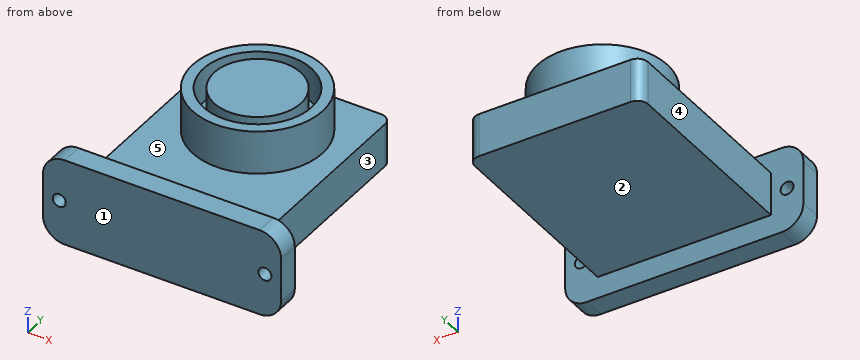
```python
from build123d import *

# Parameters (mm, degrees)
SKETCH1_W           = 40
SKETCH1_H           = 70
BOSS_EXTRUDE1_DEPTH = 10
SKETCH4_R           = 15
BOSS_EXTRUDE3_DEPTH = 10
SKETCH5_R           = 12.5
SKETCH5_R_2         = 10
CUT_EXTRUDE2_DEPTH  = 8
SKETCH6_W           = 40
SKETCH6_H           = 10
CUT_EXTRUDE3_DEPTH  = 17.5
FILLET4_R           = 2.5
SKETCH11_R          = 1.5
SKETCH11_W          = 40
SKETCH11_H          = 10
BOSS_EXTRUDE4_DEPTH = 5


with BuildPart() as part:
    # Sketch1 → Boss-Extrude1 (new body)
    with BuildSketch(Plane.XY):
        Rectangle(SKETCH1_W, SKETCH1_H)
    extrude(amount=BOSS_EXTRUDE1_DEPTH)

    # Sketch4 → Boss-Extrude3 (add)
    with BuildSketch(Plane.XY.offset(10)):
        Circle(SKETCH4_R)
    extrude(amount=BOSS_EXTRUDE3_DEPTH)

    # Sketch5 → Cut-Extrude2 (cut)
    with BuildSketch(Plane.XY.offset(20)):
        Circle(SKETCH5_R)
        Circle(SKETCH5_R_2, mode=Mode.SUBTRACT)
    extrude(amount=-CUT_EXTRUDE2_DEPTH, mode=Mode.SUBTRACT)

    # Sketch6 → Cut-Extrude3 (cut)
    with BuildSketch(Plane(origin=(0, 35, 0), x_dir=(1, 0, 0), z_dir=(0, 1, 0))):
        with Locations((0, -5)):
            Rectangle(SKETCH6_W, SKETCH6_H)
    extrude(amount=-CUT_EXTRUDE3_DEPTH, mode=Mode.SUBTRACT)

    # Fillet4
    fillet4_edges = [part.edges().sort_by_distance(p)[0] for p in [
        (-20, 17.5, 5),
        (20, 17.5, 5),
    ]]
    fillet(fillet4_edges, radius=FILLET4_R)

    # Sketch11 → Boss-Extrude4 (add)
    with BuildSketch(Plane.XZ.offset(35)):
        with BuildLine():
            Line((-22.5, 15), (22.5, 15))
            ThreePointArc((22.5, 15), (26.035533906, 13.535533906), (27.5, 10))
            Line((27.5, 10), (27.5, 0))
            ThreePointArc((27.5, 0), (26.035533906, -3.535533906), (22.5, -5))
            Line((22.5, -5), (-22.5, -5))
            ThreePointArc((-22.5, -5), (-26.035533906, -3.535533906), (-27.5, 0))
            Line((-27.5, 0), (-27.5, 10))
            ThreePointArc((-27.5, 10), (-26.035533906, 13.535533906), (-22.5, 15))
        make_face()
        with Locations((-23.75, 5)):
            Circle(SKETCH11_R, mode=Mode.SUBTRACT)
        with Locations(Location((23.75, 5, 0), (0, 0, 180))):
            Circle(SKETCH11_R, mode=Mode.SUBTRACT)
        with Locations((0, 5)):
            Rectangle(SKETCH11_W, SKETCH11_H, mode=Mode.SUBTRACT)
    extrude(amount=-BOSS_EXTRUDE4_DEPTH)


solid = part.part
```
Can you work these out from the model? Positions are in its coordinate system, mm. Face numbers are marked on the shaded views. A direction names the side the tool comes from. Give positions to 0.01 mm unless a question says otherwise; leave off trailing zeros. Loops run counter-clockwise (first coordinate to the right, second up) from the corner with the lowest first, then second, coordinate; pieces in that order, holes last. Notation, with made-up numbers: M 76.5,24 L 115.5,24 A14 ccw 115.5,48 Z; hole C 72,83.25 d8. An arc over 180 degrees is marked long. One line per question, with ' | ' between items. Start each with the question number.
Q1. For the marked faces 1, 2, 3, 4 and 5, which set-ups out of +Z, -Z, +X, -X, +Y, -Y let a thin tool reach every point of the face, with its end or its side?
Q2. If we section it at D-D (x = -23.75): Please give me the cut outline in (y, z), plus the area to 3 significant figures.
Q3. For pin 1 Ø12 at (x, y) = (5, -11.5) entering from -Z; pin 2 Ø1.5 at (x, y) = (-11, -29) entering from +Z; pin 3 Ø5 at (x, z) = (-23.75, 5) entering from +Y, each with a flat end and sliding along its axis, tell me the tip position at first contact or that it passes through.
Q4. If we section it at C-C (y = -4.5): Please give me the cut outline in (x, z), plus the area to 3 significant figures.
Q5. If we section it at A-A (z = 5): Please give me the cut outline in (x, y).
Q6. If I drill on line 1 (X direction, y = -1.5, z = 4.25); line 2 (Y direction, x = 6.5, z = 14.5); line 3 (Z direction, x = 17, y = 7), over which ranges is the centre line in solid material (lowest first)? Write a range as from..to.
Q7. If we section it at B-B (x = 0): Please give me the cut outline in (y, z).
Computed:
1) face 1: +Z, -Z, +X, -X, -Y | face 2: -Z, +X, -X, +Y | face 3: +Z, -Z, +X, +Y | face 4: +Z, -Z, -X, +Y | face 5: +Z
2) outline: M -35,-4.84 L -30,-4.84 L -30,3.5 L -35,3.5 Z; M -35,6.5 L -30,6.5 L -30,14.84 L -35,14.84 Z | area: 83.4 mm²
3) pin 1: stops at z = 0 | pin 2: stops at z = 10 | pin 3: stops at y = -30
4) outline: M -20,0 L 20,0 L 20,10 L 14.31,10 L 14.31,20 L 11.66,20 L 11.66,12 L 8.93,12 L 8.93,20 L -8.93,20 L -8.93,12 L -11.66,12 L -11.66,20 L -14.31,20 L -14.31,10 L -20,10 Z | area: 642 mm²
5) outline: M -27.5,-35 L -25.25,-35 L -25.25,-30 L -27.5,-30 Z; M -22.25,-35 L 22.25,-35 L 22.25,-30 L 20,-30 L 20,15 A2.5 ccw 17.5,17.5 L -17.5,17.5 A2.5 ccw -20,15 L -20,-30 L -22.25,-30 Z; M 25.25,-35 L 27.5,-35 L 27.5,-30 L 25.25,-30 Z
6) line 1: x = -20..20 | line 2: y = -35..-30, -13.52..-10.68, -7.6..7.6, 10.68..13.52 | line 3: z = 0..10
7) outline: M -35,-5 L -30,-5 L -30,0 L 17.5,0 L 17.5,10 L 15,10 L 15,20 L 12.5,20 L 12.5,12 L 10,12 L 10,20 L -10,20 L -10,12 L -12.5,12 L -12.5,20 L -15,20 L -15,10 L -30,10 L -30,15 L -35,15 Z
